Build history of the part. All positions in model axes, mm. A direction names the side the tool comes from. Give positions to 0.01 mm unless a question says otherwise; leave off trailing zeros. Write each loop counter-clockwise with the first axis right and the second up, starting at its lowest first coordinate (ties: lowest second). Pieces come first, ordered by that corner, then holes. Notation, with made-up numbers: (46, 85) -> (95, 85) arc R10 cw to (95, 95) -> close; hole circle Ø3 at (66, 60.5). An arc over 180 degrees is marked (long way). Put each result on its own line as item: value. Start each with the question number.
Item 1: Slice it at C-C, the plane x = 196.5. List the corners of the cut face in (y, z), plus the area to 3 significant figures.
Item 2: Slice it at D-D, the plane x = 129.5. List the corners of the cut face in (y, z).
Item 3: Tool access for faces 4 (the cylindrical face through (175.194, 140.319, 6.787)), 5 (the cylindrical face through (173.435, 80.529, 15.913)), 6 (the cylindrical face through (177.594, 142.719, 8.282)), 7 (the flat face through (136, 55, 8)): list every direction of +Z, -Z, +X, -X, +Y, -Y with a clear straight run to the whole face (end or side of a thin tool).
Item 4: Two-plate mould, pull along X, no slides. Class faces 1 (the cylindrical face through (94.806, 140.319, 7.013)), 2 (the flat face through (180, 101, 8)), 3 (the flat face through (76, 79, 0)): pulls with the +X half, pulls with the -X half, needs draft (parallel to the pull), parting line crosses it, or undercut.
Item 5: Drill centre lines: line 1 along Y through (x, z) = (3.5, -0.5); line 2 along X through (y, z) = (151.5, -0.25); line 3 along Y through (x, z) = (122, 3). Where is each one in solid material? Low to high.
Item 6: Slice it at B-B, the plane z = 10.25. List the corners of the cut face in (x, y).
Item 7: Flat gauge pins, fed straight in: pin 1 Ø2.5 at (x, y) = (3.5, 151.5) entering from -Z; pin 2 Ø2 at (y, z) = (97.5, 16) entering from -X; pin 3 Ø9 at (x, y) = (99.5, 135.5) entering from -Z; pin 4 Ø0.5 at (x, z) = (140, 16) entering from +Y. Where does each tip first touch, or does it go through?
Item 8: Slice it at A-A, the plane y = 151.5. List the corners of the cut face in (x, z), plus the area to 3 significant figures.
Autodesk Fusion 360 part; units mm, degrees
sketch "Sketch1" plane through (0, 0, 0) normal (0, 0, 1) x (1, 0, 0)
  line L0 (0, 0) -> (200, 0)
  line L1 (200, 0) -> (200, 155)
  line L2 (200, 155) -> (0, 155)
  line L3 (0, 155) -> (0, 0)
  line L4 (135, 100) -> (135, 145) construction
  line L5 (135, 100) -> (135, 55) construction
  circle A0 centre (135, 100) radius 40 construction
  line L6 (135, 100) -> (90, 100) construction
  line L7 (135, 100) -> (180, 100) construction
  line L8 (90, 145) -> (180, 145) construction
  line L9 (180, 145) -> (180, 55) construction
  line L10 (180, 55) -> (90, 55) construction
  line L11 (90, 55) -> (90, 145) construction
  line L12 (90, 145) -> (92.4, 145) construction
  line L13 (92.4, 145) -> (92.4, 142.6) construction
  line L14 (92.4, 142.6) -> (90, 142.6) construction
  line L15 (90, 142.6) -> (90, 145) construction
  line L16 (180, 55) -> (177.6, 55) construction
  line L17 (177.6, 55) -> (177.6, 57.4) construction
  line L18 (177.6, 57.4) -> (180, 57.4) construction
  line L19 (180, 57.4) -> (180, 55) construction
  line L20 (90, 145) -> (180, 145)
  line L21 (180, 145) -> (180, 55)
  line L22 (180, 55) -> (90, 55)
  line L23 (90, 55) -> (90, 145)
  line L24 (92.4, 142.6) -> (177.6, 142.6)
  line L25 (177.6, 142.6) -> (177.6, 57.4)
  line L26 (177.6, 57.4) -> (92.4, 57.4)
  line L27 (92.4, 57.4) -> (92.4, 142.6)
  dimension "d1" = 200
  dimension "d2" = 155
  dimension "d5" = 2.4
  dimension "d6" = 2.4
  dimension "d7" = 2.4
  dimension "d8" = 2.4
extrude "Extrude1" add sketch "Sketch1" against normal blind 1.2 contours L0 L1 L2 L3 makes body 1
extrude "Extrude2" add sketch "Sketch1" along normal blind 15 separate body contours L20 L21 L22 L23 makes body 2
sketch "Sketch2" plane through (0, 0, 15) normal (0, 0, 1) x (-1, 0, 0)
  line L0 (-177.6, -57.4) -> (-92.4, -57.4)
  line L1 (-92.4, -57.4) -> (-92.4, -142.6)
  line L2 (-92.4, -142.6) -> (-177.6, -142.6)
  line L3 (-177.6, -142.6) -> (-177.6, -57.4)
  line L4 (-90, -55) -> (-180, -55)
  line L5 (-180, -55) -> (-180, -145)
  line L6 (-180, -145) -> (-90, -145)
  line L7 (-90, -145) -> (-90, -55)
  line L8 (-95, -140) -> (-99.5, -140) construction
  line L9 (-99.5, -140) -> (-99.5, -135.5) construction
  line L10 (-99.5, -135.5) -> (-95, -135.5) construction
  line L11 (-95, -135.5) -> (-95, -140) construction
  line L12 (-175, -60) -> (-170.5, -60) construction
  line L13 (-170.5, -60) -> (-170.5, -64.5) construction
  line L14 (-170.5, -64.5) -> (-175, -64.5) construction
  line L15 (-175, -64.5) -> (-175, -60) construction
  line L16 (-99.5, -135.5) -> (-170.5, -135.5) construction
  line L17 (-170.5, -135.5) -> (-170.5, -64.5) construction
  line L18 (-170.5, -64.5) -> (-99.5, -64.5) construction
  line L19 (-99.5, -64.5) -> (-99.5, -135.5) construction
  circle A0 centre (-99.5, -135.5) radius 2.75
  circle A1 centre (-170.5, -135.5) radius 2.75
  circle A2 centre (-99.5, -64.5) radius 2.75
  circle A3 centre (-170.5, -64.5) radius 2.75
  line L20 (-115, -140) -> (-95, -120)
  line L21 (-95, -120) -> (-95, -80)
  line L22 (-95, -80) -> (-115, -60)
  line L23 (-115, -60) -> (-155, -60)
  line L24 (-155, -60) -> (-175, -80)
  line L25 (-175, -80) -> (-175, -120)
  line L26 (-175, -120) -> (-155, -140)
  line L27 (-155, -140) -> (-115, -140)
  line L28 (-90, -145) -> (-180, -145)
  line L29 (-180, -145) -> (-180, -55)
  line L30 (-180, -55) -> (-90, -55)
  line L31 (-90, -55) -> (-90, -145)
  dimension "d13" = 4.5
  dimension "d14" = 4.5
  dimension "d15" = 4.5
  dimension "d16" = 4.5
  dimension "d17" = 5.5
  dimension "d18" = 5.5
  dimension "d19" = 5.5
  dimension "d20" = 5.5
extrude "Extrude3" add sketch "Sketch2" along normal blind 1.8 contours L0 L1 L2 L3 | L4 L5 L6 L7 L28 L29 L30 L31 bodies 2
fillet "Fillet1" radius 20 8 edges at (95, 80, 15.9) (115, 60, 15.9) (155, 60, 15.9) (175, 80, 15.9) (175, 120, 15.9) (155, 140, 15.9) (115, 140, 15.9) (95, 120, 15.9) on bodies 2
sketch "Sketch3" plane through (0, 0, 0) normal (0, 0, 1) x (1, 0, 0)
extrude "Extrude4" add sketch "Sketch1" against normal blind 1.2 contours L20 L21 L22 L23 bodies 1 2
fillet "Fillet2" radius 8 4 edges at (92.4, 142.6, 6.9) (177.6, 142.6, 6.9) (177.6, 57.4, 6.9) (92.4, 57.4, 6.9) on bodies 1
fillet "Fillet3" radius 8 4 edges at (90, 145, 8.4) (90, 55, 8.4) (180, 55, 8.4) (180, 145, 8.4) on bodies 1
sketch "Sketch4" plane through (0, 0, 0) normal (0, 0, 1) x (1, 0, 0)
  line L0 (200, 155) -> (196.5, 155) construction
  line L1 (196.5, 155) -> (196.5, 151.5) construction
  line L2 (196.5, 151.5) -> (200, 151.5) construction
  line L3 (200, 151.5) -> (200, 155) construction
  line L4 (0, 0) -> (3.5, 0) construction
  line L5 (3.5, 0) -> (3.5, 3.5) construction
  line L6 (3.5, 3.5) -> (0, 3.5) construction
  line L7 (0, 3.5) -> (0, 0) construction
  line L8 (3.5, 3.5) -> (196.5, 3.5) construction
  line L9 (196.5, 3.5) -> (196.5, 151.5) construction
  line L10 (196.5, 151.5) -> (3.5, 151.5) construction
  line L11 (3.5, 151.5) -> (3.5, 3.5) construction
  circle A0 centre (3.5, 151.5) radius 2.15
  circle A1 centre (3.5, 3.5) radius 2.15
  circle A2 centre (196.5, 151.5) radius 2.15
  circle A3 centre (196.5, 3.5) radius 2.15
  circle A4 centre (79.8779, 151.5) radius 2.1
  circle A5 centre (100, 3.5) radius 2.1
  dimension "d31" = 3.5
  dimension "d32" = 3.5
  dimension "d33" = 3.5
  dimension "d34" = 3.5
  dimension "d35" = 4.3
  dimension "d36" = 4.3
  dimension "d37" = 4.3
  dimension "d38" = 4.3
  dimension "d41" = 4.2
  dimension "d42" = 4.2
extrude "Extrude5" cut sketch "Sketch4" against normal blind 1.2 contours A0 | A1 | A2 | A3 bodies 1
extrude "Extrude6" cut sketch "Sketch4" against normal blind 1.2 contours A4 | A5 bodies 1
copy_body "Body->Comp1" bodies 1 removing the originals makes body 3 in component "Component"
component "Component" placed x (1, 0, 0) y (0, 1, 0) z (0, 0, 1) at (0, 0, 0)
Values follow:
1. outline: (0, -1.2) -> (1.35, -1.2) -> (1.35, 0) -> (0, 0) -> close; (5.65, -1.2) -> (149.35, -1.2) -> (149.35, 0) -> (5.65, 0) -> close; (153.65, -1.2) -> (155, -1.2) -> (155, 0) -> (153.65, 0) -> close
1. area: 176 mm2
2. outline: (0, -1.2) -> (57.4, -1.2) -> (57.4, 15) -> (60, 15) -> (60, 16.8) -> (55, 16.8) -> (55, 0) -> (0, 0) -> close; (140, 15) -> (142.6, 15) -> (142.6, -1.2) -> (155, -1.2) -> (155, 0) -> (145, 0) -> (145, 16.8) -> (140, 16.8) -> close
3. face 4: -Z
3. face 5: +Z, -Z
3. face 6: +Z, +X, +Y
3. face 7: +Z, +X, -X, -Y
4. face 1: undercut
4. face 2: pulls with the +X half
4. face 3: needs draft
5. line 1: 0 to 1.35, 5.65 to 149.35, 153.65 to 155
5. line 2: 0 to 1.35, 5.65 to 77.78, 81.98 to 194.35, 198.65 to 200
5. line 3: 55 to 57.4, 142.6 to 145
6. outline: (90, 63) arc R8 ccw to (98, 55) -> (172, 55) arc R8 ccw to (180, 63) -> (180, 137) arc R8 ccw to (172, 145) -> (98, 145) arc R8 ccw to (90, 137) -> close; hole (92.4, 65.4) arc R8 ccw to (100.4, 57.4) -> (169.6, 57.4) arc R8 ccw to (177.6, 65.4) -> (177.6, 134.6) arc R8 ccw to (169.6, 142.6) -> (100.4, 142.6) arc R8 ccw to (92.4, 134.6) -> close
7. pin 1: through
7. pin 2: x = 90
7. pin 3: z = 15
7. pin 4: y = 145
8. outline: (0, -1.2) -> (1.35, -1.2) -> (1.35, 0) -> (0, 0) -> close; (5.65, -1.2) -> (77.78, -1.2) -> (77.78, 0) -> (5.65, 0) -> close; (81.98, -1.2) -> (194.35, -1.2) -> (194.35, 0) -> (81.98, 0) -> close; (198.65, -1.2) -> (200, -1.2) -> (200, 0) -> (198.65, 0) -> close
8. area: 225 mm2
